from build123d import *

# Parameters (mm, degrees)
SALIENTE_EXTRUIR1_DEPTH    = 2
CROQUIS2_R                 = 2.05
CORTAR_EXTRUIR1_DEPTH      = 3
CROQUIS7_W                 = 60.830944854
CROQUIS7_H                 = 15
CORTAR_EXTRUIR2_DEPTH      = 1
CORTAR_EXTRUIR2_DEPTH_BACK = 5


with BuildPart() as part:
    # Croquis1 → Saliente-Extruir1 (new body)
    with BuildSketch(Plane(origin=(0, 0, 0), x_dir=(1, 0, 0), z_dir=(0, 1, 0))):
        Polygon((94, -40), (50, -40), (50, 50), (-50, 50), (-50, -40), (-94, -40), (-94, -68.768453788), (-69.76, -125.32), (69.76, -125.32), (94, -68.768453788), align=None)
    extrude(amount=SALIENTE_EXTRUIR1_DEPTH)

    # Croquis2 → Cortar-Extruir1 (cut, through all)
    with BuildSketch(Plane(origin=(0, 2, 0), x_dir=(1, 0, 0), z_dir=(0, 1, 0))):
        with Locations((-45.45, -45.45)):
            Circle(CROQUIS2_R)
        with Locations((45.45, -45.45)):
            Circle(CROQUIS2_R)
        with Locations((-45.45, 45.45)):
            Circle(CROQUIS2_R)
        with Locations((45.45, 45.45)):
            Circle(CROQUIS2_R)
    extrude(amount=-CORTAR_EXTRUIR1_DEPTH, mode=Mode.SUBTRACT)

    # Croquis7 → Cortar-Extruir2 (cut, two sides)
    with BuildSketch(Plane(origin=(0, 2, 0), x_dir=(1, 0, 0), z_dir=(0, 1, 0))) as cortar_extruir2_sk:
        Polygon((-60.845769586, -115.32), (-60.845769586, -82.66), (-68.415472427, -65), (-50.415472427, -65), (-50.415472427, -50), (-84, -50), (-84, -66.715594747), (-63.166426698, -115.32), align=None)
        with Locations((0, -57.5)):
            Rectangle(CROQUIS7_W, CROQUIS7_H)
        Polygon((84, -50), (50.415472427, -50), (50.415472427, -65), (68.415472427, -65), (60.845769586, -82.66), (60.845769586, -115.32), (63.166426698, -115.32), (84, -66.715594747), align=None)
    extrude(amount=CORTAR_EXTRUIR2_DEPTH, mode=Mode.SUBTRACT)
    extrude(cortar_extruir2_sk.sketch, amount=-CORTAR_EXTRUIR2_DEPTH_BACK, mode=Mode.SUBTRACT)


solid = part.part
Work out the finished part from the listing and answer in its coordinate system (mm). A direction names the side the tool comes from. Coordinates: 2 decimals unless noted, no trailing zeros. Write each loop counter-clockwise with the first axis right and the second up, starting at its lowest first coordinate (ties: lowest second). Pieces come first, ordered by that corner, then holes.
1. The part is cut by section C-C, the plane z = 73.5. Write down the section's boundary in (x, y).
Results list:
outline: (-91.97, 0) - (-81.09, 0) - (-81.09, 2) - (-91.97, 2) - close; (-64.77, 0) - (64.77, 0) - (64.77, 2) - (-64.77, 2) - close; (81.09, 0) - (91.97, 0) - (91.97, 2) - (81.09, 2) - close
2. Flat-ended cylindrical pins translate along their axes: pin 1 (6.5 mm diameter, centred on x = -45.45, z = 45.45, fed in from -Y); pin 2 (0.6 mm diameter, centred on x = 60.5, y = 1, fed in from -Z); pin 3 (0.6 mm diameter, centred on y = 0.5, z = 91.5, fed in from +X). Find the tip coordinate at first contact, or state that the pin passes through.
Results list:
pin 1: stops at y = 0
pin 2: stops at z = 40
pin 3: stops at x = 84.39
3. For a pull along Z with two mould halves and no side action, classify faces 3 (the flat face through (64.68, 1.01, 73.71)), 4 (the flat face through (73.437, 1.014, 91.358)), 5 (the flat face through (-1, 2, 36)), 6 (the flat face through (-82.05, 0.99, 96.65)) as +Z half, -Z half, draft (parallel to the pull), parting line (faces both ways), or undercut.
Results list:
face 3: undercut
face 4: undercut
face 5: draft
face 6: +Z half
4. For faces 1 (the flat face through (-1, 0, 36)), 2 (the flat face through (-73.73, 1.01, 90.68)), determine the directions among +Z, -Z, +X, -X, +Y, -Y from which every point of the face is accessible in a straight line to the end or side of a thin tool.
Results list:
face 1: +Z, -Z, +X, -X, -Y
face 2: +Y, -Y
5. The part is cut by section D-D, the plane z = -15.5. Write down the section's boundary in (x, y).
Results list:
outline: (-50, 0) - (50, 0) - (50, 2) - (-50, 2) - close
6. Consider line 1 along Z through (x, y) = (45.45, 0.55); line 2 along X through (y, z) = (1.65, 59); line 3 along X through (y, z) = (0.9, -45.45). Determine where each line is inside the solid, lowest interval first.
Results list:
line 1: z = -50 to -47.5, -43.4 to 43.4, 47.5 to 125.32
line 2: x = -94 to -84, -50.42 to -30.42, 30.42 to 50.42, 84 to 94
line 3: x = -50 to -47.5, -43.4 to 43.4, 47.5 to 50
7. The part is cut by section A-A, the plane y = 0.3. State how many separate pieces and enclosed holes the cut face has, and give its area (3 significant figures).
Results list:
separate pieces: 1
enclosed holes: 7
area: 20,500 mm2
8. The part is cut by section B-B, the plane x = 76. Write down the section's boundary in (y, z).
Results list:
outline: (0, 40) - (2, 40) - (2, 50) - (0, 50) - close; (0, 85.38) - (2, 85.38) - (2, 110.76) - (0, 110.76) - close
